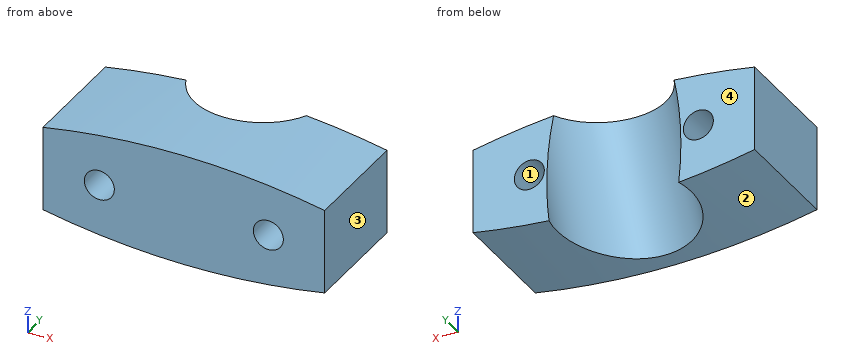
Autodesk Inventor part; units mm, degrees
ref_plane "YZ Plane" through (0, 0, 0) normal (1, 0, 0) x (0, 1, 0)
ref_plane "XZ Plane" through (0, 0, 0) normal (0, 1, 0) x (-1, 0, 0)
ref_plane "XY Plane" through (0, 0, 0) normal (0, 0, 1) x (1, 0, 0)
sketch "Sketch1" plane through (0, 0, 0) normal (0, 1, 0) x (-1, 0, 0)
  line L0 (0, 0) -> (63.5, 0)
  line L1 (63.5, 0) -> (63.5, -25.4)
  line L2 (63.5, -25.4) -> (0, -25.4)
  line L3 (0, -25.4) -> (0, 0)
  dimension "d0" = 63.5
  dimension "d1" = 25.4
extrude "Extrusion1" add sketch "Sketch1" along normal blind 26.1938
sketch "Sketch2" plane through (0, 0, 0) normal (0, -1, 0) x (1, 0, 0)
  line L0 (-63.5, 0) -> (0, 0)
  line L1 (-31.75, 0) -> (-31.75, -25.4) construction
  line L2 (0, -25.4) -> (-63.5, -25.4)
  circle A0 centre (-50.8, -12.7) radius 4.7004
  circle A1 centre (-12.7, -12.7) radius 4.7004
  dimension "d4" = 19.05
  dimension "d5" = 12.7
hole "Hole1" at (-12.7, 0, -12.7) at (-50.8, 0, -12.7) direction (0, 1, 0) diameter 6.7564 end through all
ref_plane "Work Plane6" through (-63.5, 25.0611, -27.764) normal (0, -0.4321, -0.9018) x (-1, 0, 0)
ref_plane "Work Plane5" through (-63.5, 26.1938, -25.4) normal (0, -0.4321, -0.9018) x (-1, 0, 0)
sketch "Sketch10" plane through (-63.5, 25.0611, -27.764) normal (0, -0.4321, -0.9018) x (-1, 0, 0)
  circle A0 centre (-31.75, -4.826) radius 15.113
  line L0 (-63.5, 0) -> (0, 0)
  point P0 (-63.5, -34.5974)
  dimension "d50" = 30.226
  dimension "d51" = 4.826
extrude "Extrusion9" cut sketch "Sketch10" along normal mid plane 76.2
sketch "Sketch6" plane through (0, 0, 0) normal (0, -1, 0) x (1, 0, 0)
  line L0 (0, 0) -> (-63.5, 0)
  circle A0 centre (-31.75, -165.1) radius 165.1
  line L1 (-63.5, -25.4) -> (-63.5, 0)
  line L2 (-63.5, 0) -> (-63.5, -3.0816)
  line L3 (0, 0) -> (0, -3.0816)
  line L4 (0, 0) -> (0, -25.4)
  dimension "d28" = 330.2
  dimension "d29" = 165.1
extrude "Extrusion5" cut sketch "Sketch6" against normal blind 50.8 contours L3 A0 L0 | A0 L1 L0
sketch "Sketch7" plane through (0, 0, 0) normal (0, -1, 0) x (1, 0, 0)
  line L0 (-63.5, -25.4) -> (0, -25.4) construction
  line L1 (-31.75, -25.4) -> (-31.75, 139.7) construction
  line L2 (-31.75, -25.4) -> (133.35, -25.4) construction
  circle A0 centre (-31.75, 139.7) radius 165.1
  line L3 (0, 0) -> (0, -25.4)
  line L4 (0, -22.3184) -> (0, -25.4)
  line L5 (0, -25.4) -> (-63.5, -25.4)
  line L6 (-63.5, -25.4) -> (-63.5, -22.3184)
  line L7 (-63.5, -25.4) -> (-63.5, 0)
  point P0 (0, -3.0816)
  point P1 (-63.5, -3.0816)
  dimension "d32" = 165.1
  dimension "d33" = 90
extrude "Extrusion6" cut sketch "Sketch7" against normal blind 50.8 contours A0 L5 L6 | L3 L5 A0
sketch "Sketch11" plane through (0, 26.1938, 0) normal (0, 1, 0) x (1, 0, 0)
  line L0 (8.9616, -13.4203) -> (-66.3152, -13.4203)
  line L1 (-66.3152, -13.4203) -> (-66.3152, 46.0555)
  line L2 (-66.3152, 46.0555) -> (8.9616, 46.0555)
  line L3 (8.9616, 46.0555) -> (8.9616, -13.4203)
  point P0 (0, 0)
extrude "Extrusion10" cut sketch "Sketch11" against normal blind 0.7937
properties part number "wedgeBlock"
For this review, take the finished solid that the model builds, in its own axes (mm). Face numbers are marked on the shaded views. Round coordinates to 2 decimals unless told otherwise and drop trailing zeros. Loops run counter-clockwise (first coordinate to the right, second up) from the corner with the lowest first, then second, coordinate; pieces in that order, holes last.
Q1. Mouldability with a two-part tool opening along X and no side actions: class the marked faces 1, 2, 3 and 4 as +X half, -X half, draft (parallel to the pull), parting line (faces both ways), or undercut.
Result sheet:
face 1: undercut
face 2: parting line
face 3: +X half
face 4: draft
Q2. Add section A-A on x = -12.7. Write out the cut boundary in (y, z).
Result sheet:
outline: (0, -24.3) - (25.4, -24.3) - (25.4, -16.08) - (0, -16.08) - close; (0, -9.32) - (25.4, -9.32) - (25.4, -1.1) - (0, -1.1) - close
Q3. Insertion check: pin 1 Ø3 at (x, y) = (-11.5, 20) entering from -Z; pin 2 Ø8 at (x, y) = (-44.5, 9) entering from +Z; pin 3 Ø4 at (x, z) = (-12.7, -12.7) entering from -Y; pin 4 Ø4 at (x, y) = (-18, 8) entering from +Z. Each pin has a flat end and moves straight along its axis. Give the tip position at first contact, or say it passes through.
Result sheet:
pin 1: stops at z = -24.33
pin 2: stops at z = -0.23
pin 3: passes through
pin 4: stops at z = -0.42
Q4. Add section B-B on z = -12.7. Give the number of separate pieces and of enclosed holes in the cut face, plus the area to 3 significant figures.
Result sheet:
separate pieces: 3
enclosed holes: 0
area: 918 mm2
Q5. To check wall thickness, follow line 1 along X through (y, z) = (6.5, -12.7); line 2 along X through (y, z) = (15.25, -12.7); line 3 along X through (y, z) = (13.5, -12.7). State the ranges of each line that lie inside material, in increasing order.
Result sheet:
line 1: x = -63.5 to -54.18, -47.42 to -16.08, -9.32 to 0
line 2: x = -63.5 to -54.18, -47.42 to -42.59, -20.91 to -16.08, -9.32 to 0
line 3: x = -63.5 to -54.18, -47.42 to -40.79, -22.71 to -16.08, -9.32 to 0
